For this review, use the dimensioned drawing (mm, ordinates from the lowest corner) and the shaded views. Round coordinates to 2 decimals unless told otherwise and drop trailing zeros. Write each loop counter-clockwise with the first axis right and the second up, starting at its lowest first coordinate (ties: lowest second). Pieces come first, ordered by that corner, then holes. Notation, with made-up numbers: (70, 52) -> (127, 52) arc R21 cw to (127, 89) -> close; hole circle Ø2 at (44, 53.25). An arc over 180 degrees is marked (long way). Write each question's results on one line, items separated by ' | '. Start each with the question number.
Item 1: Add section C-C (y = 8.25). State the section outline as (x, z) points, plus the area to 3 significant figures.
Item 2: To check wall thickness, follow line 1 along Y through (x, z) = (5, 5); line 2 along X through (y, z) = (1, 2); line 3 along Y through (x, z) = (4, 3). State the ranges of each line that lie inside material, in increasing order.
Item 3: Add section B-B (z = 6.75). State the section outline as (x, y) points.
Item 4: Clearance check with flat-ended pins moving along their axes: pin 1 (3 mm diameter, centred on x = 1.5, z = 4, fed in from +Y); pin 2 (4 mm diameter, centred on y = 7.5, z = 3, fed in from +X) (1 decimal); pin 3 (5 mm diameter, centred on x = 4, z = 4.5, fed in from +Y); pin 4 (5 mm diameter, centred on x = 8, z = 7, fed in from -Y) (1 decimal). State where each tip first meets the part, or that it passes through.
Item 5: Add section A-A (y = 5). State the section outline as (x, z) points.
Item 6: The part is to be moulded in two halves that separate along Y. For the marked faces 1, 2 and 3, say which applies: +Y half, -Y half, draft (parallel to the pull), parting line (faces both ways), or undercut.
Item 7: Add section D-D (x = 6.75). State the section outline as (y, z) points.
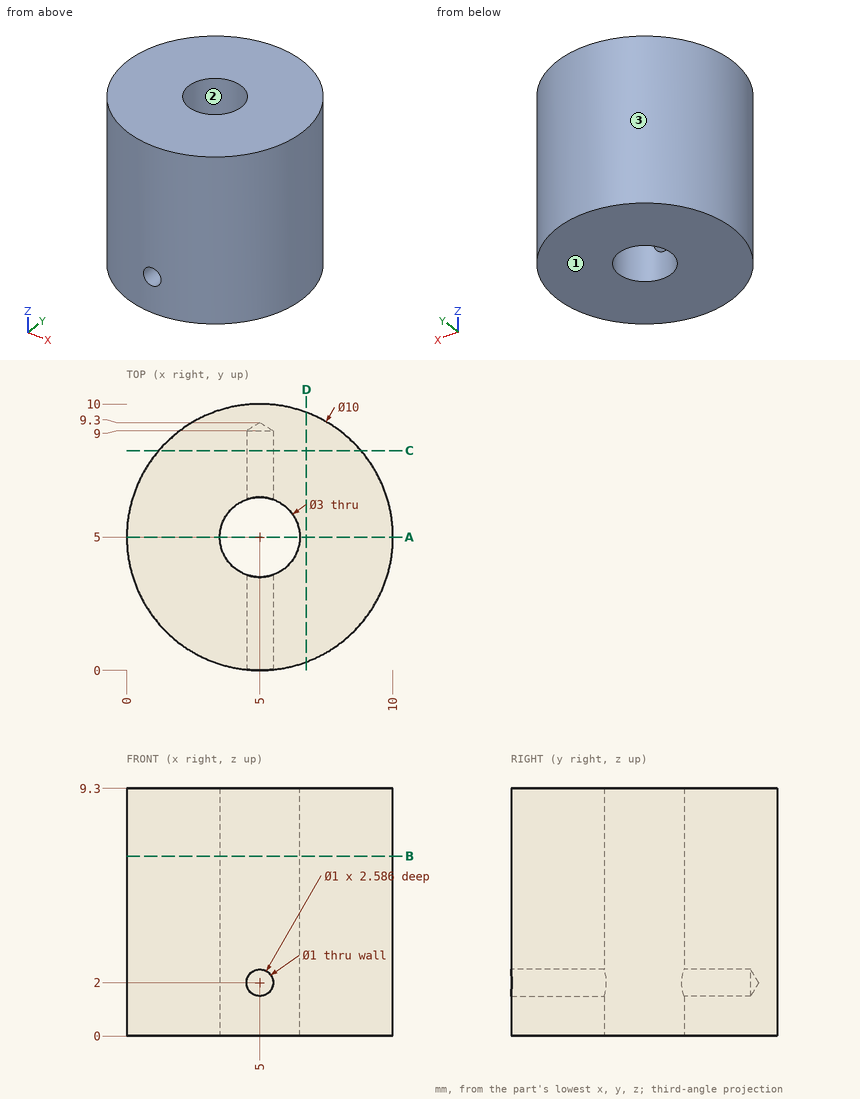
Responses:
1) outline: (1.2, 0) -> (8.8, 0) -> (8.8, 9.3) -> (1.2, 9.3) -> close; hole circle Ø1 at (5, 2) | area: 69.9 mm^2
2) line 1: y = 0 to 3.5, 6.5 to 10 | line 2: x = 2 to 4.5, 5.5 to 8 | line 3: y = 0.1 to 3.88, 6.12 to 9.9
3) outline: circle Ø10 at (5, 5); hole circle Ø3 at (5, 5)
4) pin 1: stops at y = 9.58 | pin 2: stops at x = 10 | pin 3: stops at y = 10 | pin 4: stops at y = 0
5) outline: (0, 0) -> (3.5, 0) -> (3.5, 9.3) -> (0, 9.3) -> close; (6.5, 0) -> (10, 0) -> (10, 9.3) -> (6.5, 9.3) -> close
6) face 1: draft | face 2: undercut | face 3: parting line
7) outline: (0.32, 0) -> (9.68, 0) -> (9.68, 9.3) -> (0.32, 9.3) -> close
